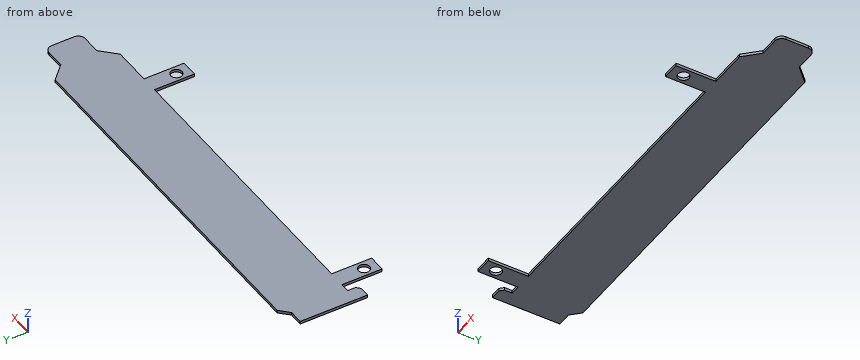
```python
from build123d import *

# Parameters (mm, degrees)
F0_W     = 4.801906
F0_H     = 11.323674
F0_R     = 1.5875
F1_DEPTH = 0.8


with BuildPart() as f1:
    # F0 (on Top) → F1 (new body)
    with BuildSketch(Plane.XY):
        with BuildLine():
            ThreePointArc((120.0679, -6.0198), (119.509938, -4.672762), (118.1629, -4.1148))
            Line((118.1629, -4.1148), (112.7506, -4.1148))
            Line((112.7506, -4.1148), (108.6358, 0))
            Line((108.6358, 0), (6.477, 0))
            Line((6.477, 0), (3.937, -2.54))
            Line((3.937, -2.54), (0, -2.54))
            Line((0, -2.54), (0, -18.415))
            Line((0, -18.415), (0, -21.59))
            Line((0, -21.59), (2.921, -21.59))
            Line((2.921, -21.59), (3.937, -20.574))
            Line((3.937, -20.574), (3.937, -18.415))
            Line((3.937, -18.415), (6.552547, -18.415))
            Line((6.552547, -18.415), (11.354453, -18.415))
            Line((11.354453, -18.415), (92.912547, -18.415))
            Line((92.912547, -18.415), (97.714453, -18.415))
            Line((97.714453, -18.415), (108.6358, -18.415))
            Line((108.6358, -18.415), (112.7506, -14.3002))
            Line((112.7506, -14.3002), (118.1629, -14.3002))
            ThreePointArc((118.1629, -14.3002), (119.509938, -13.742238), (120.0679, -12.3952))
            Line((120.0679, -12.3952), (120.0679, -6.0198))
        make_face()
        with Locations((8.9535, -24.076837)):
            Rectangle(F0_W, F0_H)
        with Locations((8.9535, -26.0985)):
            Circle(F0_R, mode=Mode.SUBTRACT)
        with Locations((95.3135, -24.076837)):
            Rectangle(F0_W, F0_H)
        with Locations((95.3135, -26.0985)):
            Circle(F0_R, mode=Mode.SUBTRACT)
    extrude(amount=F1_DEPTH)


solid = f1.part
```
Input: part model. Units: mm. Frame: model coordinates. Round coordinates to 2 decimals unless told otherwise and drop trailing zeros. Write each loop counter-clockwise with the first axis right and the second up, starting at its lowest first coordinate (ties: lowest second). Pieces come first, ordered by that corner, then holes. Notation, with made-up numbers: (-16.5, 56.5) -> (6.5, 56.5) arc R25 ccw to (6.5, 83.5) -> close; hole circle Ø4 at (-28, 88). An arc over 180 degrees is marked (long way). Answer as CSV lines item,"result".
1. Section A-A (z = 0.6). Return the cut outline in (x, y) (1 decimal).
Geometry says:
outline,"(0, -21.6) -> (2.9, -21.6) -> (3.9, -20.6) -> (3.9, -18.4) -> (6.6, -18.4) -> (6.6, -29.7) -> (11.4, -29.7) -> (11.4, -18.4) -> (92.9, -18.4) -> (92.9, -29.7) -> (97.7, -29.7) -> (97.7, -18.4) -> (108.6, -18.4) -> (112.8, -14.3) -> (118.2, -14.3) arc R1.9 ccw to (120.1, -12.4) -> (120.1, -6) arc R1.9 ccw to (118.2, -4.1) -> (112.8, -4.1) -> (108.6, 0) -> (6.5, 0) -> (3.9, -2.5) -> (0, -2.5) -> close; hole circle Ø3.2 at (9, -26.1); hole circle Ø3.2 at (95.3, -26.1)"
2. Section B-B (x = 19.5). Return the cut outline in (y, z) (3 decimals), plus the area to 3 significant figures.
Geometry says:
outline,"(-18.415, 0) -> (0, 0) -> (0, 0.8) -> (-18.415, 0.8) -> close"
area,"14.7 mm^2"
3. Ray query, L1, parallel to X at y = -26.25, z = 0.75; L2, parallel to X at y = -18.5, z = 0.3; L3, parallel to Y at x = 67, z = 0.2 (3 decimals). Return the intervals inside material, ascending. Write a range as [from, to].
Geometry says:
L1,"x = [6.55, 7.37], [10.53, 11.35], [92.91, 93.73], [96.89, 97.71]"
L2,"x = [0, 3.94], [6.55, 11.35], [92.91, 97.71]"
L3,"y = [-18.415, 0]"
4. Contact query for a flat-ended pin moving along its axis: P1, Ø3, axis at x = 8.95, y = -26.1, coming from the +Z side. Output: stop coordinate, or through.
Geometry says:
P1,"passes through"
